```python
from build123d import *

# Parameters (mm, degrees)
SKETCH1_R           = 2.32
SKETCH1_R_2         = 2
SKETCH1_R_3         = 5
SKETCH1_R_4         = 23
SKETCH1_R_5         = 1.5
SKETCH1_W           = 8
SKETCH1_H           = 35
SKETCH1_W_2         = 20
SKETCH1_H_2         = 8
BOSS_EXTRUDE1_DEPTH = 4
FILLET1_R           = 30
FILLET2_R           = 20


with BuildPart() as part:
    # Sketch1 → Boss-Extrude1 (new body)
    with BuildSketch(Plane(origin=(0, 0, 0), x_dir=(1, 0, 0), z_dir=(0, 1, 0))):
        Polygon((-153.14810061, 75), (-117.14810061, 75), (-117.14810061, -75), (-153.14810061, -75), (-153.14810061, -90), (56.85189939, -90), (56.85189939, -75), (20.85189939, -75), (20.85189939, 75), (56.85189939, 75), (56.85189939, 90), (20.85189939, 90), (-7.14810061, 90), (-7.14810061, 80), (-7.14810061, 60), (-89.14810061, 60), (-89.14810061, 73), (-89.14810061, 90), (-129.14810061, 90), (-153.14810061, 90), align=None)
        with Locations(Location((-128.14810061, -80, 0), (0, 0, 270))):
            Circle(SKETCH1_R, mode=Mode.SUBTRACT)
        with Locations(Location((-128.14810061, 80, 0), (0, 0, 90))):
            Circle(SKETCH1_R, mode=Mode.SUBTRACT)
        with Locations(Location((31.85189939, 80, 0), (0, 0, 270))):
            Circle(SKETCH1_R, mode=Mode.SUBTRACT)
        with Locations(Location((31.85189939, -80, 0), (0, 0, 90))):
            Circle(SKETCH1_R, mode=Mode.SUBTRACT)
        with Locations(Location((-108.14810061, -48, 0), (0, 0, 270))):
            Circle(SKETCH1_R_2, mode=Mode.SUBTRACT)
        with Locations(Location((-92.14810061, -48, 0), (0, 0, 270))):
            Circle(SKETCH1_R_2, mode=Mode.SUBTRACT)
        with Locations(Location((-92.14810061, -32, 0), (0, 0, 90))):
            Circle(SKETCH1_R_2, mode=Mode.SUBTRACT)
        with Locations(Location((-108.14810061, -32, 0), (0, 0, 90))):
            Circle(SKETCH1_R_2, mode=Mode.SUBTRACT)
        with Locations(Location((-100.14810061, -40, 0), (0, 0, 270))):
            Circle(SKETCH1_R_3, mode=Mode.SUBTRACT)
        with Locations(Location((-92.14810061, 48, 0), (0, 0, 90))):
            Circle(SKETCH1_R_2, mode=Mode.SUBTRACT)
        with Locations(Location((-108.14810061, 48, 0), (0, 0, 90))):
            Circle(SKETCH1_R_2, mode=Mode.SUBTRACT)
        with Locations(Location((-92.14810061, 32, 0), (0, 0, 270))):
            Circle(SKETCH1_R_2, mode=Mode.SUBTRACT)
        with Locations(Location((-100.14810061, 40, 0), (0, 0, 90))):
            Circle(SKETCH1_R_3, mode=Mode.SUBTRACT)
        with Locations(Location((-108.14810061, 32, 0), (0, 0, 270))):
            Circle(SKETCH1_R_2, mode=Mode.SUBTRACT)
        with Locations(Location((-4.14810061, -32, 0), (0, 0, 270))):
            Circle(SKETCH1_R_2, mode=Mode.SUBTRACT)
        with Locations(Location((-4.14810061, -48, 0), (0, 0, 90))):
            Circle(SKETCH1_R_2, mode=Mode.SUBTRACT)
        with Locations(Location((3.85189939, -40, 0), (0, 0, 90))):
            Circle(SKETCH1_R_3, mode=Mode.SUBTRACT)
        with Locations(Location((11.85189939, -48, 0), (0, 0, 90))):
            Circle(SKETCH1_R_2, mode=Mode.SUBTRACT)
        with Locations(Location((11.85189939, -32, 0), (0, 0, 270))):
            Circle(SKETCH1_R_2, mode=Mode.SUBTRACT)
        with Locations(Location((-4.14810061, 32, 0), (0, 0, 90))):
            Circle(SKETCH1_R_2, mode=Mode.SUBTRACT)
        with Locations(Location((-4.14810061, 48, 0), (0, 0, 270))):
            Circle(SKETCH1_R_2, mode=Mode.SUBTRACT)
        with Locations(Location((11.85189939, 32, 0), (0, 0, 90))):
            Circle(SKETCH1_R_2, mode=Mode.SUBTRACT)
        with Locations(Location((11.85189939, 48, 0), (0, 0, 270))):
            Circle(SKETCH1_R_2, mode=Mode.SUBTRACT)
        with Locations(Location((3.85189939, 40, 0), (0, 0, 270))):
            Circle(SKETCH1_R_3, mode=Mode.SUBTRACT)
        with Locations(Location((-48.14810061, 0, 0), (0, 0, 270))):
            Circle(SKETCH1_R_4, mode=Mode.SUBTRACT)
        with Locations(Location((-93.14810061, 67.5, 0), (0, 0, 270))):
            Circle(SKETCH1_R_5, mode=Mode.SUBTRACT)
        with Locations(Location((-3.14810061, 67.5, 0), (0, 0, 90))):
            Circle(SKETCH1_R_5, mode=Mode.SUBTRACT)
        with Locations(Location((-61.24810061, 49.5, 0), (0, 0, 270))):
            Circle(SKETCH1_R_5, mode=Mode.SUBTRACT)
        with Locations(Location((-35.04810061, 49.5, 0), (0, 0, 90))):
            Circle(SKETCH1_R_5, mode=Mode.SUBTRACT)
        with Locations(Location((-73.14810061, -45, 0), (0, 0, 270))):
            Circle(SKETCH1_R_2, mode=Mode.SUBTRACT)
        with Locations(Location((-23.14810061, -45, 0), (0, 0, 90))):
            Circle(SKETCH1_R_2, mode=Mode.SUBTRACT)
        with Locations(Location((9.85189939, 61, 0), (0, 0, 270))):
            Circle(SKETCH1_R_2, mode=Mode.SUBTRACT)
        with Locations(Location((-106.14810061, 61, 0), (0, 0, 90))):
            Circle(SKETCH1_R_2, mode=Mode.SUBTRACT)
        with Locations((-105.14810061, -2.5)):
            Rectangle(SKETCH1_W, SKETCH1_H, mode=Mode.SUBTRACT)
        with Locations((8.85189939, -2.5)):
            Rectangle(SKETCH1_W, SKETCH1_H, mode=Mode.SUBTRACT)
        with Locations((-48.14810061, 36)):
            Rectangle(SKETCH1_W_2, SKETCH1_H_2, mode=Mode.SUBTRACT)
    extrude(amount=BOSS_EXTRUDE1_DEPTH)

    # Fillet1
    # the kernel refuses this fillet: 30 mm, written as the material it takes off along each edge
    with BuildSketch(Plane(origin=(-153.14810061, -64.951905284, -90), x_dir=(1, 0, 0), z_dir=(0, 1, 0))) as fillet1_piece_1:
        with BuildLine():
            CenterArc((25.980762114, -30), FILLET1_R, 90, 60)
            Line((0, -15), (-0.519615242, -14.7))
            ThreePointArc((-0.519615242, -14.7), (-0.6, -7.5), (-0.6, 0))
            Line((-0.6, 0), (0, 0.6))
            Line((0, 0.6), (25.980762114, 0.6))
            Line((25.980762114, 0.6), (25.980762114, 0))
        make_face()
    extrude(amount=133.903810568, mode=Mode.SUBTRACT)
    with BuildSketch(Plane(origin=(56.85189939, -64.951905284, -90), x_dir=(-1, 0, 0), z_dir=(0, 1, 0))) as fillet1_piece_2:
        with BuildLine():
            CenterArc((25.980762114, 30), FILLET1_R, 210, 60)
            Line((0, 15), (-0.519615242, 14.7))
            ThreePointArc((-0.519615242, 14.7), (-0.6, 7.5), (-0.6, 0))
            Line((-0.6, 0), (0, -0.6))
            Line((0, -0.6), (25.980762114, -0.6))
            Line((25.980762114, -0.6), (25.980762114, 0))
        make_face()
    extrude(amount=133.903810568, mode=Mode.SUBTRACT)

    # Fillet2
    # the kernel refuses this fillet: 20 mm, written as the material it takes off along each edge
    with BuildSketch(Plane(origin=(56.85189939, -48.412291828, 90), x_dir=(0, 0, -1), z_dir=(0, 1, 0))) as fillet2_piece_1:
        with BuildLine():
            CenterArc((20, 19.364916731), FILLET2_R, 180, 75.522487814)
            Line((0, 19.364916731), (-0.4, 19.364916731))
            Line((-0.4, 19.364916731), (-0.4, 0))
            Line((-0.4, 0), (0, -0.4))
            ThreePointArc((0, -0.4), (7.5, -0.4), (14.9, -0.387298335))
            Line((14.9, -0.387298335), (15, 0))
        make_face()
    extrude(amount=100.824583655, mode=Mode.SUBTRACT)
    with BuildSketch(Plane(origin=(-153.14810061, -48.412291828, 90), x_dir=(1, 0, 0), z_dir=(0, 1, 0))) as fillet2_piece_2:
        with BuildLine():
            CenterArc((19.364916731, 20), FILLET2_R, 194.477512186, 75.522487814)
            Line((0, 15), (-0.387298335, 14.9))
            ThreePointArc((-0.387298335, 14.9), (-0.4, 7.5), (-0.4, 0))
            Line((-0.4, 0), (0, -0.4))
            Line((0, -0.4), (19.364916731, -0.4))
            Line((19.364916731, -0.4), (19.364916731, 0))
        make_face()
    extrude(amount=100.824583655, mode=Mode.SUBTRACT)


solid = part.part
```
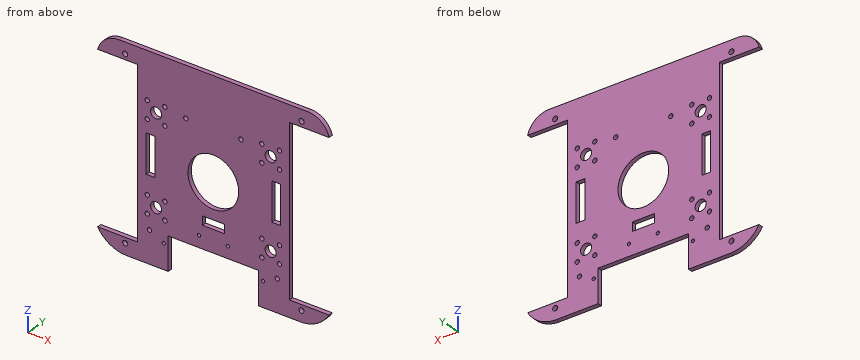
Work out the finished part from the listing and answer in its coordinate system (mm). Round coordinates to 2 decimals unless told otherwise and drop trailing zeros. Write each loop counter-clockwise with the first axis right and the second up, starting at its lowest first coordinate (ties: lowest second). Pieces come first, ordered by that corner, then holes.
1) A cutting plane is placed at C-C on y = 2.1. Give the number of separate pieces and of enclosed holes in the cut face, and give its area (3 significant figures).
2) Consider probe 1 along X at (y, z) = (3, 32); probe 2 along X at (y, z) = (1.05, 0); probe 3 along X at (y, z) = (0.85, -67.5). Determine where each line is inside the solid, lowest interval first.
3) A cutting plane is placed at A-A on z = 0. Determine the outline of the cut face in (x, y), and give its area (3 significant figures).
4) A cutting plane is placed at D-D on x = -77.5. Determine the outline of the cut face in (y, z).
5) Flat-ended cylindrical pins translate along their axes: P1, Ø3.5, axis at x = 11.85, z = 32, coming from the -Y side; P2, Ø1.5, axis at y = 1.5, z = -40, coming from the -X side; P3, Ø1.5, axis at y = 3, z = 57.5, coming from the +X side; P4, Ø8, axis at x = -100, z = -67.5, coming from the -Y side. Find the tip coordinate at first contact, or state that the pin passes through.
6) A cutting plane is placed at B-B on z = 80. Determine the outline of the cut face in (x, y).
Entries:
1. separate pieces: 1
1. enclosed holes: 36
1. area: 21,100 mm2
2. probe 1: x = -117.15 to -110.15, -106.15 to -94.15, -90.15 to -6.15, -2.15 to 9.85, 13.85 to 20.85
2. probe 2: x = -117.15 to -109.15, -101.15 to -71.15, -25.15 to 4.85, 12.85 to 20.85
2. probe 3: x = -117.15 to -94.65, -91.65 to -89.15, -7.15 to -4.65, -1.65 to 20.85
3. outline: (-117.15, 0) - (-109.15, 0) - (-109.15, 4) - (-117.15, 4) - close; (-101.15, 0) - (-71.15, 0) - (-71.15, 4) - (-101.15, 4) - close; (-25.15, 0) - (4.85, 0) - (4.85, 4) - (-25.15, 4) - close; (12.85, 0) - (20.85, 0) - (20.85, 4) - (12.85, 4) - close
3. area: 304 mm2
4. outline: (0, -60) - (4, -60) - (4, 90) - (0, 90) - close
5. P1: passes through
5. P2: stops at x = -117.15
5. P3: stops at x = 20.85
5. P4: stops at y = 0
6. outline: (-151.1, 0) - (-130.47, 0) - (-130.47, 4) - (-151.1, 4) - close; (-125.83, 0) - (29.53, 0) - (29.53, 4) - (-125.83, 4) - close; (34.17, 0) - (54.81, 0) - (54.81, 4) - (34.17, 4) - close
